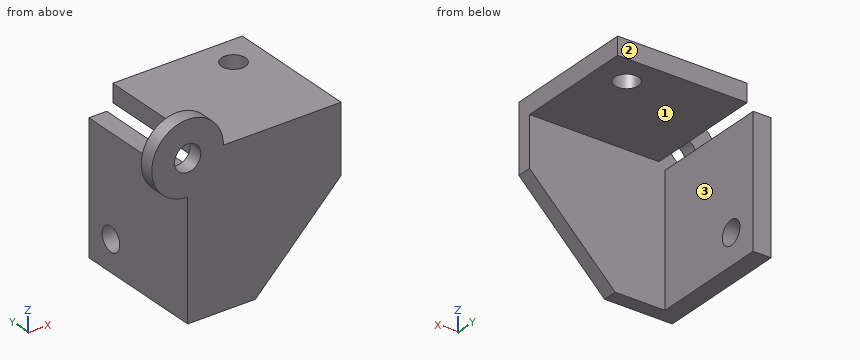
from build123d import *

# Parameters (mm, degrees)
BOSS_EXTRUDE1_DEPTH     = 5
BOSS_EXTRUDE2_DEPTH     = 15
SKETCH3_R               = 2
CUT_EXTRUDE1_DEPTH      = 34.496268449
SKETCH4_R               = 2
CUT_EXTRUDE2_DEPTH      = 34.496268449
FILLET1_R               = 1
BOSS_EXTRUDE3_DEPTH     = 2.4
BOSS_EXTRUDE4_DEPTH     = 20
CUT_EXTRUDE3_DEPTH      = 51.527220387
CUT_EXTRUDE3_DEPTH_BACK = 51.527220387
SKETCH7_R               = 2
CUT_EXTRUDE4_DEPTH      = 51.527220387
CUT_EXTRUDE4_DEPTH_BACK = 51.527220387
SKETCH8_R               = 2
CUT_EXTRUDE5_DEPTH      = 20
CUT_EXTRUDE6_DEPTH      = 32.914256521
CUT_EXTRUDE7_DEPTH      = 32.914256521
SKETCH12_R              = 6
BOSS_EXTRUDE5_DEPTH     = 2.4
CUT_EXTRUDE8_DEPTH      = 31.915717398
CUT_EXTRUDE8_DEPTH_BACK = 31.915717398
SKETCH13_R              = 2.2
SKETCH14_R              = 4
CUT_EXTRUDE9_DEPTH      = 31.915717398
CUT_EXTRUDE10_DEPTH     = 31.915717398


with BuildPart() as part:
    # Sketch1 → Boss-Extrude1 (new body)
    with BuildSketch(Plane(origin=(0, 0, 0), x_dir=(1, 0, 0), z_dir=(0, 1, 0))):
        Polygon((0, 0), (0, 19), (19, 0), align=None)
    extrude(amount=BOSS_EXTRUDE1_DEPTH)

    # Sketch2 → Boss-Extrude2 (add)
    with BuildSketch(Plane(origin=(0, 5, 0), x_dir=(1, 0, 0), z_dir=(0, 1, 0))):
        Polygon((0, 19), (0, 0), (19, 0), (16, 3), (3, 3), (3, 16), align=None)
    extrude(amount=BOSS_EXTRUDE2_DEPTH)

    # Sketch3 → Cut-Extrude1 (cut, through all)
    with BuildSketch(Plane.XY):
        with Locations((11.5, 15)):
            Circle(SKETCH3_R)
    extrude(amount=-CUT_EXTRUDE1_DEPTH, mode=Mode.SUBTRACT)

    # Sketch4 → Cut-Extrude2 (cut, through all)
    with BuildSketch(Plane.ZY):
        with Locations((-11.5, 15)):
            Circle(SKETCH4_R)
    extrude(amount=-CUT_EXTRUDE2_DEPTH, mode=Mode.SUBTRACT)

    # Fillet1
    fillet1_edges = [part.edges().sort_by_distance(p)[0] for p in [
        (9.5, 20, -3),
        (3, 20, -9.5),
        (1.5, 20, -17.5),
        (17.5, 20, -1.5),
        (19, 10, 0),
        (0, 10, -19),
    ]]
    fillet(fillet1_edges, radius=FILLET1_R)

    # Sketch5 → Boss-Extrude3 (add)
    with BuildSketch(Plane.XZ):
        Polygon((28, 9), (-9, 9), (-9, -28), align=None)
    extrude(amount=BOSS_EXTRUDE3_DEPTH)

    # Sketch6 → Boss-Extrude4 (add)
    with BuildSketch(Plane(origin=(0, 0, 0), x_dir=(1, 0, 0), z_dir=(0, 1, 0))):
        Polygon((-9, -9), (-9, 16.673246444), (-6, 16.673246444), (-6, -6), (16.666866389, -6), (16.666866389, -9), align=None)
    extrude(amount=BOSS_EXTRUDE4_DEPTH)

    # Sketch7 → Cut-Extrude3 (cut, two sides: drawn at the far end of the back side and taken through both)
    with BuildSketch(Plane.XY.offset(9).offset(-CUT_EXTRUDE3_DEPTH_BACK)):
        with Locations((11.5, 15)):
            Circle(SKETCH7_R)
    extrude(amount=CUT_EXTRUDE3_DEPTH + CUT_EXTRUDE3_DEPTH_BACK, mode=Mode.SUBTRACT)

    # Sketch8 → Cut-Extrude4 (cut, two sides: drawn at the far end of the back side and taken through both)
    with BuildSketch(Plane.ZY.offset(9).offset(-CUT_EXTRUDE4_DEPTH_BACK)):
        with Locations((-11.5, 15)):
            Circle(SKETCH8_R)
    extrude(amount=CUT_EXTRUDE4_DEPTH + CUT_EXTRUDE4_DEPTH_BACK, mode=Mode.SUBTRACT)

    # Sketch9 → Cut-Extrude5 (cut)
    with BuildSketch(Plane(origin=(0, 0, 0), x_dir=(1, 0, 0), z_dir=(0, 1, 0))):
        with BuildLine():
            Line((16.666866389, -6), (16.666866389, -9))
            Line((16.666866389, -9), (28, -9))
            Line((28, -9), (17.292893219, 1.707106781))
            ThreePointArc((17.292893219, 1.707106781), (17.524431974, 0.655116604), (16.666866389, 0.003292399))
            Line((16.666866389, 0.003292399), (16.666866389, -6))
        make_face()
        with BuildLine():
            Line((-6, 16.673246444), (0.003831968, 16.673246444))
            ThreePointArc((0.003831968, 16.673246444), (0.658123366, 17.525531279), (1.707106781, 17.292893219))
            Line((1.707106781, 17.292893219), (-9, 28))
            Line((-9, 28), (-9, 16.673246444))
            Line((-9, 16.673246444), (-6, 16.673246444))
        make_face()
    extrude(amount=-CUT_EXTRUDE5_DEPTH, mode=Mode.SUBTRACT)

    # Sketch10 → Cut-Extrude6 (cut, through all)
    with BuildSketch(Plane(origin=(0, 0, 0), x_dir=(1, 0, 0), z_dir=(0, 1, 0))):
        with BuildLine():
            Line((1.707106781, 17.292893219), (17.292893219, 1.707106781))
            ThreePointArc((17.292893219, 1.707106781), (17.50966597, 0.617316568), (16.585786438, 0))
            Line((16.585786438, 0), (0, 0))
            Line((0, 0), (0, 16.585786438))
            ThreePointArc((0, 16.585786438), (0.617316568, 17.50966597), (1.707106781, 17.292893219))
        make_face()
    extrude(amount=CUT_EXTRUDE6_DEPTH, mode=Mode.SUBTRACT)

    # Sketch11 → Cut-Extrude7 (cut, through all)
    with BuildSketch(Plane(origin=(0, 0, 0), x_dir=(1, 0, 0), z_dir=(0, 1, 0))):
        with BuildLine():
            Line((2.326753556, 16.673246444), (0.003831968, 16.673246444))
            ThreePointArc((0.003831968, 16.673246444), (0.658123366, 17.525531279), (1.707106781, 17.292893219))
            Line((1.707106781, 17.292893219), (2.326753556, 16.673246444))
        make_face()
        with BuildLine():
            Line((17.292893219, 1.707106781), (16.666866389, 2.333133611))
            Line((16.666866389, 2.333133611), (16.666866389, 0.003292399))
            ThreePointArc((16.666866389, 0.003292399), (17.524431974, 0.655116604), (17.292893219, 1.707106781))
        make_face()
    extrude(amount=-CUT_EXTRUDE7_DEPTH, mode=Mode.SUBTRACT)

    # Sketch12 → Boss-Extrude5 (add)
    with BuildSketch(Plane.XZ.offset(2.4)):
        with Locations((-9, 9)):
            Circle(SKETCH12_R)
    extrude(amount=-BOSS_EXTRUDE5_DEPTH)

    # Sketch13 → Cut-Extrude8 (cut, two sides: drawn at the far end of the back side and taken through both)
    with BuildSketch(Plane(origin=(0, 0, 0), x_dir=(1, 0, 0), z_dir=(0, 1, 0)).offset(-CUT_EXTRUDE8_DEPTH_BACK)):
        with Locations(Location((-9, -9, 0), (0, 0, 270))):
            Circle(SKETCH13_R)
    extrude(amount=CUT_EXTRUDE8_DEPTH + CUT_EXTRUDE8_DEPTH_BACK, mode=Mode.SUBTRACT)

    # Sketch14 → Cut-Extrude9 (cut, through all)
    with BuildSketch(Plane(origin=(0, 0, 0), x_dir=(1, 0, 0), z_dir=(0, 1, 0))):
        with Locations((-9, -9)):
            Circle(SKETCH14_R)
    extrude(amount=CUT_EXTRUDE9_DEPTH, mode=Mode.SUBTRACT)

    # Sketch15 → Cut-Extrude10 (cut, through all)
    with BuildSketch(Plane(origin=(0, 0, 0), x_dir=(1, 0, 0), z_dir=(0, 1, 0))):
        with BuildLine():
            Line((-9, -5), (-5, -5))
            Line((-5, -5), (-5, -9))
            ThreePointArc((-5, -9), (-6.171572875, -6.171572875), (-9, -5))
        make_face()
    extrude(amount=CUT_EXTRUDE10_DEPTH, mode=Mode.SUBTRACT)


solid = part.part
The listing builds one solid part. Answer for the finished solid, in the listing's coordinates (mm). Face numbers are marked on the shaded views. A direction names the side the tool comes from. Give positions to 0.01 mm unless a question says otherwise; leave off trailing zeros. Loops run counter-clockwise (first coordinate to the right, second up) from the corner with the lowest first, then second, coordinate; pieces in that order, holes last.
Item 1: A cutting plane is placed at A-A (y = 15). Give the vertices of the cut face in (x, z), then the cut area to 3 significant figures.
Derived:
outline: (-9, -16.67) - (-6, -16.67) - (-6, -13.5) - (-9, -13.5) - close; (-9, -9.5) - (-6, -9.5) - (-6, 5) - (-9, 5) - close; (-5, 6) - (9.5, 6) - (9.5, 9) - (-5, 9) - close; (13.5, 6) - (16.67, 6) - (16.67, 9) - (13.5, 9) - close
area: 106 mm2
Item 2: Find the intervals of material crossed by line 1 along Z through (x, y) = (-7.85, 15); line 2 along Y through (x, z) = (-2.5, -4); line 3 along Y through (x, z) = (11.5, 6.95), in increasing order.
Derived:
line 1: z = -16.67 to -13.5, -9.5 to 5
line 2: y = -2.4 to 0
line 3: y = -2.4 to 13, 17 to 20
Item 3: Each of these flat-tipped pins is pushed along its axis until it touches: pin 1 Ø11 at (y, z) = (12, -10.5) entering from -X; pin 2 Ø5 at (x, z) = (-9, 9) entering from +Y; pin 3 Ø3.5 at (y, z) = (12, 7) entering from -X; pin 4 Ø2.5 at (x, y) = (11.5, 15) entering from +Z. Where does it stop, or does it pass through?
Derived:
pin 1: stops at x = -9
pin 2: stops at y = 0
pin 3: stops at x = -5
pin 4: passes through
Item 4: A cutting plane is placed at B-B (x = 11.5). Give the vertices of the cut face in (y, z), then the cut area to 3 significant figures.
Derived:
outline: (-2.4, -7.5) - (0, -7.5) - (0, 6) - (13, 6) - (13, 9) - (-2.4, 9) - close; (17, 6) - (20, 6) - (20, 9) - (17, 9) - close
area: 87.6 mm2
Item 5: A tool of negligible diameter and unlimited length cuts with its end or side. For the marked faces 1, 2 and 3, from which of +Z, -Z, +X, -X, +Y, -Y can it reach the whole face along a straight path? Write none if from no direction.
Derived:
face 1: -Z, +X, -X, +Y
face 2: +Z, -Z, +X, -X, +Y
face 3: +Z, -Z, +X, +Y
Item 6: A cutting plane is placed at C-C (y = -0.75). Give the vertices of the cut face in (x, z), then the cut area to 3 significant figures.
Derived:
outline: (-9, -16.67) - (2.33, -16.67) - (16.67, -2.33) - (16.67, 9) - (-3, 9) arc R6 ccw (long way) to (-9, 3) - close; hole circle Ø4.4 at (-9, 9)
area: 626 mm2
Item 7: A cutting plane is placed at D-D (z = -10). Give the vertices of the cut face in (x, y).
Derived:
outline: (-9, -2.4) - (9, -2.4) - (9, 0) - (-6, 0) - (-6, 13.68) - (-9, 13.68) - close; (-9, 16.32) - (-6, 16.32) - (-6, 20) - (-9, 20) - close
